Drawing for the job (mm, zero at the part's lowest x, y, z). A direction names the side the tool comes from. Give positions to 0.01 mm unless a question says otherwise; leave off trailing zeros. Order: outer loops, then holes, each group sorted by start corner. A loop starts at its lowest first (then second) coordinate and runs counter-clockwise, first axis right, second up. Notation, with made-up numbers: (-25, -34.5) - (-20, -34.5) arc R25 ccw to (-20, -11.5) - close; hole circle Ø8 at (88.25, 79). An arc over 180 degrees is marked (long way). Use a Markdown table: item, result.
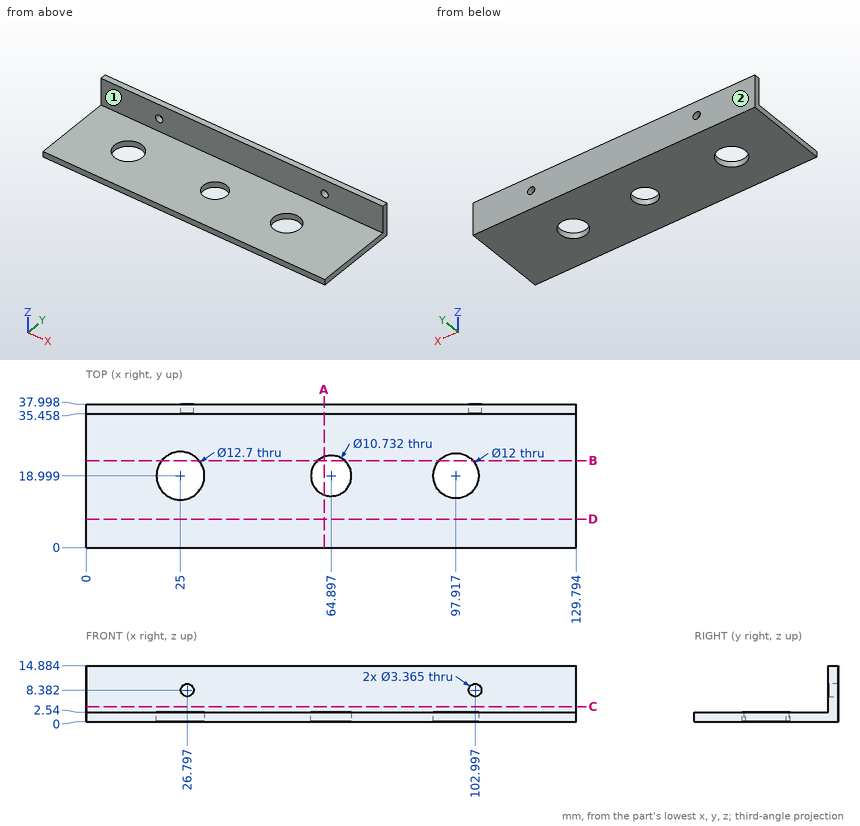
1) Slice it at D-D (y = 7.5). Write the cut outline in (x, z) (1 decimal).
Computed:
| item | result |
|---|---|
| outline | (0, 0) - (129.8, 0) - (129.8, 2.5) - (0, 2.5) - close |
2) Slice it at A-A (x = 63). Write the cut outline in (y, z) (1 decimal), and give its area (3 significant figures).
Computed:
| item | result |
|---|---|
| outline | (0, 0) - (14, 0) - (14, 2.5) - (0, 2.5) - close; (24, 0) - (38, 0) - (38, 14.9) - (35.5, 14.9) - (35.5, 2.5) - (24, 2.5) - close |
| area | 102 mm² |
3) Tool access for the marked faces 1 and 2: list every direction of +Z, -Z, +X, -X, +Y, -Y with a clear straight run to the whole face (end or side of a thin tool).
Computed:
| item | result |
|---|---|
| face 1 | +Z, +X, -X, -Y |
| face 2 | +Z, -Z, +X, -X, +Y |
4) Slice it at B-B (y = 23). Write the cut outline in (x, z) (1 decimal), and give its area (3 significant figures).
Computed:
| item | result |
|---|---|
| outline | (0, 0) - (20.1, 0) - (20.1, 2.5) - (0, 2.5) - close; (29.9, 0) - (61.3, 0) - (61.3, 2.5) - (29.9, 2.5) - close; (68.5, 0) - (93.4, 0) - (93.4, 2.5) - (68.5, 2.5) - close; (102.4, 0) - (129.8, 0) - (129.8, 2.5) - (102.4, 2.5) - close |
| area | 264 mm² |
5) Pin check, flat tips, straight feed: P1, Ø10.5, axis at x = 56, y = 21, coming from the +Z side; P2, Ø6, axis at x = 73, z = 11, coming from the -Y side. Stop position of each tip, or through.
Computed:
| item | result |
|---|---|
| P1 | stops at z = 2.54 |
| P2 | stops at y = 35.46 |
6) Wall check: line 1 (X direction, y = 23, z = 2.5) (1 decimal); line 2 (Y direction, x = 25.5, z = 0.5); line 3 (Z direction, x = 107, y = 24). Give the ranges that are in metal, low to high. Write a range as from..to.
Computed:
| item | result |
|---|---|
| line 1 | x = 0..20.1, 29.9..61.3, 68.5..93.4, 102.4..129.8 |
| line 2 | y = 0..12.67, 25.33..38 |
| line 3 | z = 0..2.54 |
7) Slice it at C-C (z = 4). Write the cut outline in (x, y) (1 decimal).
Computed:
| item | result |
|---|---|
| outline | (0, 35.5) - (129.8, 35.5) - (129.8, 38) - (0, 38) - close |
